Can you work these out from the model? Positions are in its coordinate system, mm. A direction names the side the tool comes from. Give positions to 0.01 mm unless a question says otherwise; leave off trailing zeros. Loops run counter-clockwise (first coordinate to the right, second up) from the corner with the lowest first, then second, coordinate; pieces in that order, holes last. Notation, with made-up numbers: (-17.75, 48) - (-1.75, 48) arc R21 cw to (-1.75, 62) - close; hole circle Ø10 at (33.5, -35). An arc over 180 degrees is marked (long way). Answer as a JSON object with one key per item and string values.
```python
from build123d import *

# Parameters (mm, degrees)
F1_DEPTH = 4
F2_DEPTH = 2
F3_START = 2
F3_DEPTH = 2
F4_SIZE  = 1.99999
F5_R     = 2
F6_DEPTH = 3.75
F7_DEPTH = 3.5
F8_DEPTH = 3.25
F9_DEPTH = 3


# Not quite as in the source:
# - a fillet or chamfer is up to 0.001 mm smaller than in the source, because OpenCascade refuses the exact size


with BuildPart() as f1:
    # F0 (on Top) → F1 (new body)
    with BuildSketch(Plane.XY):
        Polygon((32.7846783229, 14.824549064), (4.8026783229, 63.2907947614), (-23.1793216771, 14.824549064), align=None)
        Polygon((-19.715220062, 16.824549064), (4.8026783229, 59.2907947614), (29.3205767077, 16.824549064), align=None, mode=Mode.SUBTRACT)
    extrude(amount=F1_DEPTH)

    # F0 (on Top) → F2 (join)
    with BuildSketch(Plane.XY):
        Polygon((37.1148053418, 12.324549064), (4.8026783229, 68.2907947614), (-27.509448696, 12.324549064), align=None)
        Polygon((-23.1793216771, 14.824549064), (4.8026783229, 63.2907947614), (32.7846783229, 14.824549064), align=None, mode=Mode.SUBTRACT)
    extrude(amount=F2_DEPTH)

    # F0 (on Top) → F3 (join)
    with BuildSketch(Plane.XY.offset(F3_START)):
        Polygon((29.3205767077, 16.824549064), (4.8026783229, 59.2907947614), (-19.715220062, 16.824549064), align=None)
    extrude(amount=F3_DEPTH)

    # F4 (size 2 in the source; OpenCascade refuses exactly that, so slightly less here)
    f4_edges = [f1.edges().sort_by_distance(p)[0] for p in [
        (4.802678, 16.824549, 0),
        (-7.456271, 38.057672, 0),
        (17.061628, 38.057672, 0),
    ]]
    chamfer(f4_edges, length=F4_SIZE)

    # F5 (on face) → F6 (cut)
    with BuildSketch(Plane.XY):
        with BuildLine():
            Line((15.8012454512, 40.2407176847), (14.8071694273, 41.9625078646))
            ThreePointArc((14.8071694273, 41.9625078646), (12.0675004242, 39.2368445398), (15.801257126, 40.2338840067))
            ThreePointArc((15.801257126, 40.2338840067), (15.8012542073, 40.2373008507), (15.8012454512, 40.2407176847))
        make_face()
        with Locations((-10.6723830104, 23.3052875847)):
            Circle(F5_R)
    extrude(amount=F6_DEPTH, mode=Mode.SUBTRACT)

    # F5 (on face) → F7 (cut)
    with BuildSketch(Plane.XY):
        with BuildLine():
            Line((3.6860700174, 34.755180139), (9.4204377363, 37.8238173116))
            ThreePointArc((9.4204377363, 37.8238173116), (9.2694965624, 38.1212680469), (9.1387235678, 38.4281207834))
            Line((9.1387235678, 38.4281207834), (0.9941436583, 35.2838113904))
            Line((0.9941436583, 35.2838113904), (-2.8154677711, 33.8130667806))
            Line((-2.8154677711, 33.8130667806), (1.0452440474, 33.3419926465))
            Line((1.0452440474, 33.3419926465), (3.6860700174, 34.755180139))
        make_face()
        with BuildLine():
            Line((17.0693753854, 23.8813530259), (14.9441122519, 35.3662478082))
            ThreePointArc((14.9441122519, 35.3662478082), (14.2087911946, 35.2505200844), (13.4644377158, 35.2452416378))
            Line((13.4644377158, 35.2452416378), (12.8494622186, 26.1368211359))
            Line((12.8494622186, 26.1368211359), (15.8132929355, 24.552706629))
            Line((15.8132929355, 24.552706629), (17.0693753854, 23.8813530259))
        make_face()
        with BuildLine():
            Line((-13.4587365793, 16.824549064), (-6.1025659626, 16.824549064))
            Line((-6.1025659626, 16.824549064), (-3.819498702, 19.0105444595))
            Line((-3.819498702, 19.0105444595), (-1.2189327972, 21.5005390346))
            Line((-1.2189327972, 21.5005390346), (-7.725601985, 22.742720621))
            ThreePointArc((-7.725601985, 22.742720621), (-9.2656609828, 20.6555454959), (-11.8573356204, 20.5492238495))
            Line((-11.8573356204, 20.5492238495), (-13.4587365793, 16.824549064))
        make_face()
        with BuildLine():
            ThreePointArc((9.6781818277, 43.0623553402), (10.154568974, 43.6546537332), (10.7152328484, 44.1678964823))
            Line((10.7152328484, 44.1678964823), (5.5434275419, 50.7608279586))
            Line((5.5434275419, 50.7608279586), (5.1609951292, 49.6271412781))
            Line((5.1609951292, 49.6271412781), (4.2115291581, 46.8125343323))
            Line((4.2115291581, 46.8125343323), (9.6781818277, 43.0623553402))
        make_face()
    extrude(amount=F7_DEPTH, mode=Mode.SUBTRACT)

    # F5 (on face) → F8 (cut)
    with BuildSketch(Plane.XY):
        with BuildLine():
            Line((19.8564007878, 24.4885329157), (15.5959561349, 35.5670804467))
            ThreePointArc((15.5959561349, 35.5670804467), (15.2734627879, 35.4555359146), (14.9441122519, 35.3662478082))
            Line((14.9441122519, 35.3662478082), (17.0693753854, 23.8813530259))
            Line((17.0693753854, 23.8813530259), (15.8132929355, 24.552706629))
            Line((15.8132929355, 24.552706629), (17.4690298736, 20.0315453112))
            Line((17.4690298736, 20.0315453112), (19.8564007878, 24.4885329157))
        make_face()
        Polygon((-6.1025659626, 16.824549064), (1.2875116271, 16.824549064), (1.7734020948, 17.1169545501), (-3.819498702, 19.0105444595), align=None)
        with BuildLine():
            Line((5.785849411, 33.66388008), (9.9342960343, 37.064244924))
            ThreePointArc((9.9342960343, 37.064244924), (9.6599157648, 37.4322252607), (9.4204377363, 37.8238173116))
            Line((9.4204377363, 37.8238173116), (3.6860700174, 34.755180139))
            Line((3.6860700174, 34.755180139), (5.785849411, 33.66388008))
        make_face()
        with BuildLine():
            ThreePointArc((11.5326481984, 44.6896009562), (11.8941525727, 44.8558913869), (12.2677356256, 44.9929082563))
            Line((12.2677356256, 44.9929082563), (11.2701070238, 48.0888796571))
            Line((11.2701070238, 48.0888796571), (7.7075759005, 54.2593645662))
            Line((7.7075759005, 54.2593645662), (6.1958078295, 55.1715530455))
            Line((6.1958078295, 55.1715530455), (7.7216781624, 52.1746300315))
            Line((7.7216781624, 52.1746300315), (11.5326481984, 44.6896009562))
        make_face()
        with BuildLine():
            ThreePointArc((-12.7082549566, 21.1018299793), (-12.079105038, 25.9550296735), (-7.7066088949, 23.7571547066))
            Line((-7.7066088949, 23.7571547066), (-6.6805827438, 23.5612770993))
            ThreePointArc((-6.6805827438, 23.5612770993), (-12.5480123805, 26.8382770364), (-13.1208381636, 20.1422088056))
            Line((-13.1208381636, 20.1422088056), (-12.7082549566, 21.1018299793))
        make_face()
    extrude(amount=F8_DEPTH, mode=Mode.SUBTRACT)

    # F5 (on face) → F9 (cut)
    with BuildSketch(Plane.XY):
        with BuildLine():
            ThreePointArc((9.1387235678, 38.4281207834), (8.9697402045, 38.9468547775), (8.8582790135, 39.4809116441))
            Line((8.8582790135, 39.4809116441), (1.4540485572, 38.196541369))
            Line((1.4540485572, 38.196541369), (0.9941436583, 35.2838113904))
            Line((0.9941436583, 35.2838113904), (9.1387235678, 38.4281207834))
        make_face()
        with BuildLine():
            ThreePointArc((10.7152328484, 44.1678964823), (11.1112630591, 44.4486119837), (11.5326481984, 44.6896009562))
            Line((11.5326481984, 44.6896009562), (7.7216781624, 52.1746300315))
            Line((7.7216781624, 52.1746300315), (3.6355266348, 51.2855537236))
            Line((3.6355266348, 51.2855537236), (5.1609951292, 49.6271412781))
            Line((5.1609951292, 49.6271412781), (5.5434275419, 50.7608279586))
            Line((5.5434275419, 50.7608279586), (10.7152328484, 44.1678964823))
        make_face()
    extrude(amount=F9_DEPTH, mode=Mode.SUBTRACT)


solid = f1.part
```
1) Imagine slicing it at B-B on z = 1. Write out the boundary of the cut face in (x, y).
Check sheet entries:
{"outline": "(-27.51, 12.32) - (37.11, 12.32) - (4.8, 68.29) - close; hole (-21.45, 15.82) - (31.05, 15.82) - (4.8, 61.29) - close"}
2) Which directions (+Z, -Z, +X, -X, +Y, -Y) give clear straight access to the entire face, cutting with the end or side of a thin tool? Please do faces 4 (the flat face through (21.185, 39.916, 0.986)), 5 (the flat face through (8, 49, 3)).
Check sheet entries:
{"face 4": "+Z, -Z, +X, +Y", "face 5": "-Z"}
3) If we mould it in two halves opening along Y, with no side actions, what happens to faces 1 (the flat face through (-11.127, 40.699, 0.986)), 2 (the flat face through (-11, 23, 3.75)), 3 (the flat face through (4, 34, 4))? For each: released by +Y, released by -Y, zero draft, split by the parting line, or undercut.
Check sheet entries:
{"face 1": "released by +Y", "face 2": "undercut", "face 3": "zero draft"}
4) I need wall thicknesses on L1, parallel to X at y = 21, z = 2.85; L2, parallel to Y at x = 21, z = 3.3; L3, parallel to X at y = 49.5, z = 3.3. Which ranges of each line are inside material? Lowest first, please.
Check sheet entries:
{"L1": "-19.61 to -13.94, -12.75 to -8.75, -1.74 to 17.11, 17.99 to 29.22", "L2": "14.82 to 35.24", "L3": "-3.16 to 5.12, 6.53 to 12.76"}
5) I'm going to push flat-ended pins straight in: P1, Ø3.5, axis at x = 16, y = 30, coming from the -Z side; P2, Ø2, axis at x = 13.5, y = 40.5, coming from the -Z side; P3, Ø1.8, axis at x = -5, y = 19.5, coming from the -Z side; P4, Ø12, axis at x = 18.5, y = 48.5, coming from the +Z side. Where does each tip first touch, or does it pass through?
Check sheet entries:
{"P1": "z = 2", "P2": "z = 3.75", "P3": "z = 3.5", "P4": "z = 4"}
